Design review of the part built by this model. Coordinates are the model's own, in mm. A direction names the side the tool comes from. Give positions to 0.01 mm unless a question says otherwise; leave off trailing zeros. Loops run counter-clockwise (first coordinate to the right, second up) from the corner with the lowest first, then second, coordinate; pieces in that order, holes last.
from build123d import *

# Parameters (mm, degrees)
BOSS_EXTRUDE1_DEPTH = 250
SHELL1_T            = -2
SKETCH2_W           = 31
SKETCH2_H           = 31
CUT_EXTRUDE1_DEPTH  = 259.843582111


with BuildPart() as part:
    # Sketch1 → Boss-Extrude1 (new, symmetric)
    with BuildSketch(Plane(origin=(0, 0, 0), x_dir=(1, 0, 0), z_dir=(0, 1, 0))):
        with BuildLine():
            Line((-24, -30), (24, -30))
            ThreePointArc((24, -30), (28.242640687, -28.242640687), (30, -24))
            Line((30, -24), (30, 24))
            ThreePointArc((30, 24), (28.242640687, 28.242640687), (24, 30))
            Line((24, 30), (-24, 30))
            ThreePointArc((-24, 30), (-28.242640687, 28.242640687), (-30, 24))
            Line((-30, 24), (-30, -24))
            ThreePointArc((-30, -24), (-28.242640687, -28.242640687), (-24, -30))
        make_face()
    extrude(amount=BOSS_EXTRUDE1_DEPTH, both=True)

    # Shell1
    shell1_openings = [part.faces().sort_by_distance(p)[0] for p in [
        (0, 250, 0),
        (0, -250, 0),
    ]]
    offset(amount=SHELL1_T, openings=shell1_openings, kind=Kind.INTERSECTION)

    # Sketch2 → Cut-Extrude1 (cut, through all)
    with BuildSketch(Plane(origin=(0, 0, -30), x_dir=(-1, 0, 0), z_dir=(0, 0, -1))):
        with Locations((0, 3.002147222)):
            Rectangle(SKETCH2_W, SKETCH2_H)
    extrude(amount=-CUT_EXTRUDE1_DEPTH, mode=Mode.SUBTRACT)


solid = part.part
Q1. Take a section at C-C (y = 149.5). Give the boundary of the cut face in (x, z).
Results:
outline: (-30, -24) arc R6 ccw to (-24, -30) - (24, -30) arc R6 ccw to (30, -24) - (30, 24) arc R6 ccw to (24, 30) - (-24, 30) arc R6 ccw to (-30, 24) - close; hole (-28, -24) arc R4 ccw to (-24, -28) - (24, -28) arc R4 ccw to (28, -24) - (28, 24) arc R4 ccw to (24, 28) - (-24, 28) arc R4 ccw to (-28, 24) - close
Q2. Draft analysis for pull direction Z (two halves, no side actions). For faces 3 (the face through (28, 4, 0)), 4 (the face through (-16, 4, -30)), 5 (the face through (0, 250, -29)), state which applies: pulls with the +Z half, pulls with the -Z half, needs draft (parallel to the pull), parting line crosses it, or undercut.
Results:
face 3: undercut
face 4: pulls with the -Z half
face 5: needs draft
Q3. Insertion check: pin 1 (10 mm diameter, centred on x = -22, z = -1, fed in from +Y); pin 2 (1 mm diameter, centred on y = 3, z = 28.5, fed in from -X); pin 3 (1.6 mm diameter, centred on y = -1, z = -29.5, fed in from -X); pin 4 (2 mm diameter, centred on y = 5.5, z = 29, fed in from +X). Each pin has a flat end and moves straight along its axis. Give the tip position at first contact, or say it passes through.
Results:
pin 1: passes through
pin 2: stops at x = -28.47
pin 3: stops at x = -27.73
pin 4: stops at x = 28.47
Q4. Take a section at B-B (z = -1). Give the boundary of the cut face in (x, y).
Results:
outline: (-30, -250) - (-28, -250) - (-28, 250) - (-30, 250) - close; (28, -250) - (30, -250) - (30, 250) - (28, 250) - close
Q5. Tool access review of faces 1 (the face through (-30, 4, 0)), 2 (the face through (-28, 4, 0)): name each direction out of +Z, -Z, +X, -X, +Y, -Y from which nothing blocks a thin tool from reaching the whole face with its end or side.
Results:
face 1: +Z, -Z, -X, +Y, -Y
face 2: +Y, -Y
Q6. Wall thickness on line 1 (X direction, y = -124.5, z = -23.5); line 2 (Z direction, x = -27.5, y = 128): over which ranges is each line inside the solid? List them lowest first.
Results:
line 1: x = -30 to -28, 28 to 30
line 2: z = -28.87 to -25.94, 25.94 to 28.87
Q7. Take a section at A-A (x = -4.5). Give the boundary of the cut face in (y, z).
Results:
outline: (-250, -30) - (-12.5, -30) - (-12.5, -28) - (-250, -28) - close; (-250, 28) - (-12.5, 28) - (-12.5, 30) - (-250, 30) - close; (18.5, -30) - (250, -30) - (250, -28) - (18.5, -28) - close; (18.5, 28) - (250, 28) - (250, 30) - (18.5, 30) - close
